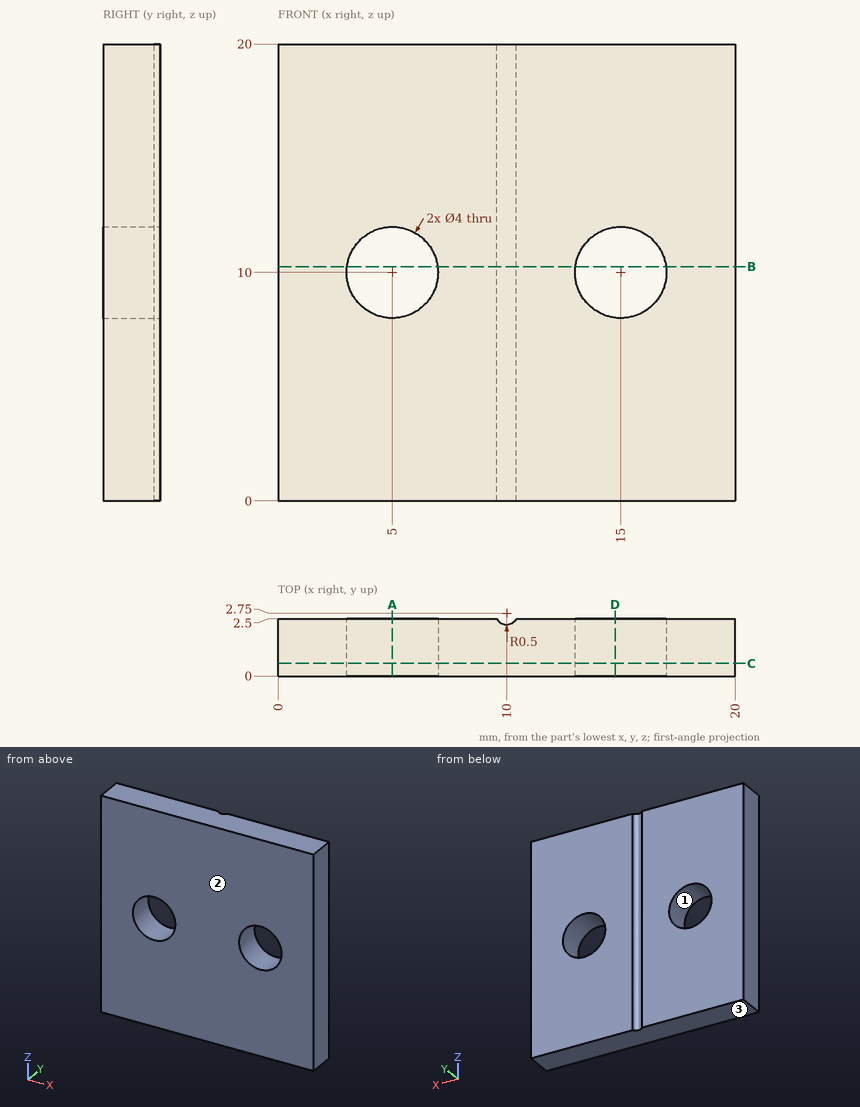
Study the drawing (mm; zero at the part's minimum x, y, z) and answer. Round coordinates to 2 decimals unless told otherwise and drop trailing zeros. Loops run counter-clockwise (first coordinate to the right, second up) from the corner with the lowest first, then second, coordinate; pieces in that order, holes last.
Q1. Section B-B, the plane z = 10.25 is taken. Determine the outline of the cut face in (x, y).
Q2. Section A-A, the plane x = 5 is taken. Determine the outline of the cut face in (y, z).
Q3. Find the intervals of material crossed by line 1 (X direction, y = 0.9, z = 10); line 2 (Z direction, x = 15, y = 2.05); line 3 (X direction, y = 1.65, z = 8.25), in increasing order.
Q4. Section D-D, the plane x = 14.75 is taken. Determine the outline of the cut face in (y, z).
Q5. Section C-C, the plane y = 0.55 is taken. Determine the outline of the cut face in (x, z).
Q6. For a pull along Z with two mould halves and no side action, classify the marked faces 1, 2 and 3 as released by +Z, released by -Z, zero draft, split by the parting line, or undercut.
Completed:
1. outline: (0, 0) - (3.02, 0) - (3.02, 2.5) - (0, 2.5) - close; (6.98, 0) - (13.02, 0) - (13.02, 2.5) - (10.43, 2.5) arc R0.5 cw to (9.57, 2.5) - (6.98, 2.5) - close; (16.98, 0) - (20, 0) - (20, 2.5) - (16.98, 2.5) - close
2. outline: (0, 0) - (2.5, 0) - (2.5, 8) - (0, 8) - close; (0, 12) - (2.5, 12) - (2.5, 20) - (0, 20) - close
3. line 1: x = 0 to 3, 7 to 13, 17 to 20
3. line 2: z = 0 to 8, 12 to 20
3. line 3: x = 0 to 4.03, 5.97 to 14.03, 15.97 to 20
4. outline: (0, 0) - (2.5, 0) - (2.5, 8.02) - (0, 8.02) - close; (0, 11.98) - (2.5, 11.98) - (2.5, 20) - (0, 20) - close
5. outline: (0, 0) - (20, 0) - (20, 20) - (0, 20) - close; hole circle Ø4 at (5, 10); hole circle Ø4 at (15, 10)
6. face 1: undercut
6. face 2: zero draft
6. face 3: released by -Z
